Part model, mm, in its own coordinate system. A direction names the side the tool comes from. Round coordinates to 2 decimals unless told otherwise and drop trailing zeros. Loops run counter-clockwise (first coordinate to the right, second up) from the corner with the lowest first, then second, coordinate; pieces in that order, holes last.
1) 3-axis set-ups, long thin cutter, end or side, ignore diameter. For faces 1 (the flat face through (0, 2.25, 11)), 2 (the flat face through (0, 1.25, 11)): which of +Z, -Z, +X, -X, +Y, -Y reach the whole face in a straight line?
2) Band-saw the part on A-A, the plane y = 0.2. Write the cut outline in (x, z).
3) Drop a flat-ended pin along its axis: P1, Ø1, axis at y = 1, z = 7, coming from the -X side. Give the stop position or say it passes through.
4) Mould opens along X. For faces 3 (the flat face through (-5.148, -0.018, 14.749)), 4 (the flat face through (0, -1.25, 11)), 5 (the flat face through (0, 0, 30)) say: +X half, -X half, draft (parallel to the pull), parting line (faces both ways), or undercut.
5) Probe line 1 (Y direction, x = -2.5, z = 10.25); line 2 (Z direction, x = 0.5, y = -0.75). List the from-to ranges inside material, lowest first.
6) Band-saw the part on B-B, the plane x = 0. Write the cut outline in (y, z), then the cut area to 3 significant figures.
7) Band-saw the part on C-C, the plane y = 1.9. Write the cut outline in (x, z).
from build123d import *

# Parameters (mm, degrees)
F1_DEPTH = 2.25
F2_R     = 1
F3_T     = 1


# Not quite as in the source:
# - a shell that OpenCascade refuses in one call is made with other operations: the cavity is built on its own and cut out


with BuildPart() as f1:
    # F0 (on Front) → F1 (new body, symmetric)
    with BuildSketch(Plane.XZ):
        Polygon((-3.75, 30), (-6.5, 0), (6.5, 0), (3.75, 30), align=None)
    extrude(amount=F1_DEPTH, both=True)

    # F2
    f2_edges = [f1.edges().sort_by_distance(p)[0] for p in [
        (-3.75, 0, 30),
        (3.75, 0, 30),
        (5.125, -2.25, 15),
        (0, -2.25, 30),
        (-5.125, -2.25, 15),
        (-5.125, 2.25, 15),
        (5.125, 2.25, 15),
        (0, 2.25, 30),
    ]]
    fillet(f2_edges, radius=F2_R)

    # F3: shell of thickness 1, made by hand


with BuildPart() as f3_core1:
    # F3_t2: copy of F1
    add(f1.part)

    # the walls: a layer under each face that stays
    f3_faces = [f3_core1.faces().sort_by_distance(p)[0] for p in [
        (-5.1666494856, 0, 14.5456419748),
        (0, 2.25, 14.5),
        (0, -2.25, 14.5),
        (5.1666494856, 0, 14.5456419748),
        (0, 0, 30),
    ]]
    thicken(f3_faces, amount=-F3_T, mode=Mode.SUBTRACT)


with BuildPart() as f1_1:
    add(f1.part)

    # what is left inside the walls is the cavity
    f3_cavity = [f3_core1.part.solids().sort_by_distance(p)[0] for p in [
        (0, -1.24, 9.666667),
    ]]
    add(f3_cavity, mode=Mode.SUBTRACT)


solid = f1_1.part
Reported:
1. face 1: +Z, -Z, +X, -X, +Y
1. face 2: -Z
2. outline: (-6.5, 0) - (-5.5, 0) - (-2.84, 29) - (2.84, 29) - (5.5, 0) - (6.5, 0) - (3.83, 29.09) arc R1 ccw to (2.84, 30) - (-2.84, 30) arc R1 ccw to (-3.83, 29.09) - close
3. P1: stops at x = -5.9
4. face 3: -X half
4. face 4: undercut
4. face 5: draft
5. line 1: y = -2.25 to -1.25, 1.25 to 2.25
5. line 2: z = 29 to 30
6. outline: (-2.25, 0) - (-1.25, 0) - (-1.25, 29) - (1.25, 29) - (1.25, 0) - (2.25, 0) - (2.25, 29) arc R1 ccw to (1.25, 30) - (-1.25, 30) arc R1 ccw to (-2.25, 29) - close
6. area: 62.1 mm2
7. outline: (-6.26, 0) - (6.26, 0) - (3.59, 29.07) arc R0.76 ccw to (2.84, 29.76) - (-2.84, 29.76) arc R0.76 ccw to (-3.59, 29.07) - close
